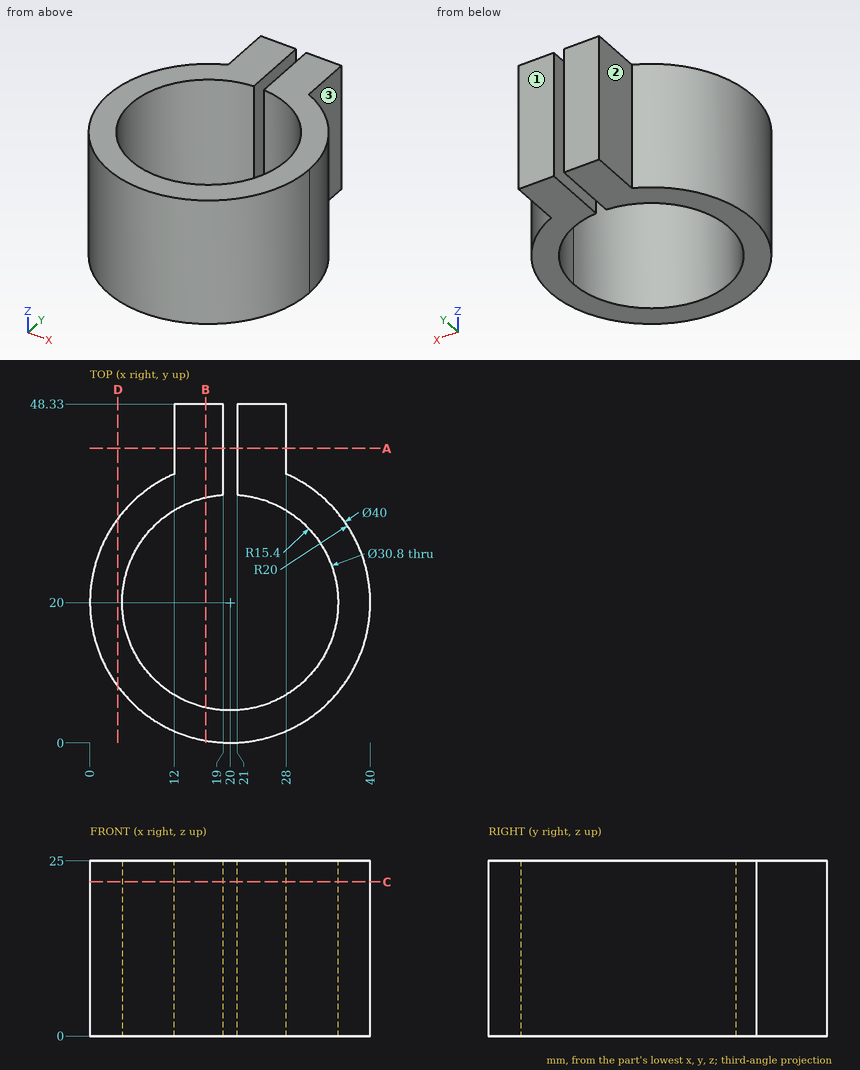
Drawing for the job (mm, zero at the part's lowest x, y, z). A direction names the side the tool comes from. Round coordinates to 2 decimals unless told otherwise and drop trailing zeros. Write each loop counter-clockwise with the first axis right and the second up, starting at its lowest first coordinate (ties: lowest second). Pieces come first, ordered by that corner, then holes.
Item 1: Tool access for the marked faces 1, 2 and 3: list every direction of +Z, -Z, +X, -X, +Y, -Y with a clear straight run to the whole face (end or side of a thin tool).
Filled in:
face 1: +Z, -Z, +X, -X, +Y
face 2: +Z, -Z, -X, +Y
face 3: +Z, -Z, +X, +Y
Item 2: Band-saw the part on A-A on y = 42. Write the cut outline in (x, z), then the cut area to 3 significant figures.
Filled in:
outline: (12, 0) - (19, 0) - (19, 25) - (12, 25) - close; (21, 0) - (28, 0) - (28, 25) - (21, 25) - close
area: 350 mm2
Item 3: Drill centre lines: L1, parallel to X at y = 43.5, z = 13; L2, parallel to Y at x = 29, z = 1 (1 decimal); L3, parallel to X at y = 16.5, z = 20. Where is each one in solid material? Low to high.
Filled in:
L1: x = 12 to 19, 21 to 28
L2: y = 2.1 to 7.5, 32.5 to 37.9
L3: x = 0.31 to 5, 35 to 39.69
Item 4: Drop flat-ended pins along their axis: pin 1 Ø6 at (x, z) = (5.5, 5.5) entering from +Y; pin 2 Ø11 at (y, z) = (41, 15.5) entering from -X; pin 3 Ø4 at (x, z) = (17.5, 20.5) entering from -Y; pin 4 Ø8 at (x, y) = (13, 26.5) entering from +Z. Give the stop position or say it passes through.
Filled in:
pin 1: stops at y = 36.36
pin 2: stops at x = 7.36
pin 3: stops at y = 0.01
pin 4: passes through
Item 5: Band-saw the part on B-B on x = 16.5. Write the cut outline in (y, z), then the cut area to 3 significant figures.
Filled in:
outline: (0.31, 0) - (5, 0) - (5, 25) - (0.31, 25) - close; (35, 0) - (48.33, 0) - (48.33, 25) - (35, 25) - close
area: 451 mm2
Item 6: Band-saw the part on D-D on x = 4. Write the cut outline in (y, z).
Filled in:
outline: (8, 0) - (32, 0) - (32, 25) - (8, 25) - close
Item 7: Band-saw the part on C-C on z = 22. Write the cut outline in (x, y), then the cut area to 3 significant figures.
Filled in:
outline: (12, 38.33) arc R20 ccw (long way) to (28, 38.33) - (28, 48.33) - (21, 48.33) - (21, 35.37) arc R15.4 cw (long way) to (19, 35.37) - (19, 48.33) - (12, 48.33) - close
area: 628 mm2
